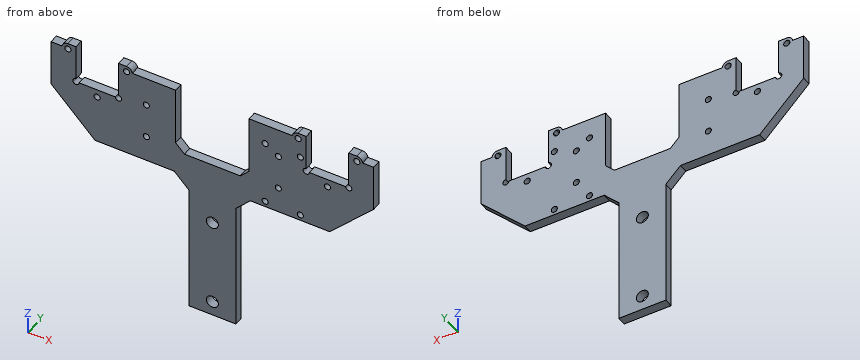
from build123d import *

# Parameters (mm, degrees)
EXTRUDE_6_DEPTH         = 3
HOLE_WIZARD_4_1_4_1_1_D = 4.1
HOLE_WIZARD_2_1_2_1_1_D = 2.1
EXTRUDE_START           = -3
SKETCH_39_R             = 1.05
EXTRUDE_7_DEPTH         = 3
HOLE_WIZARD_2_1_2_1_2_D = 2.1
CHAMFER_3_SIZE          = 3


with BuildPart() as part:
    # 草图33 → 凸台-拉伸6 (new body)
    with BuildSketch(Plane(origin=(0, 0, 0), x_dir=(1, 0, 0), z_dir=(0, 1, 0))):
        Polygon((110, 16), (110, 0), (101.5, 0), (101.5, 11.5), (87, 11.5), (87, 0), (67.5, 0), (67.5, 23), (42.5, 23), (42.5, 0), (23, 0), (23, 11.5), (8.5, 11.5), (8.5, 0), (0, 0), (0, 16), (15, 31), (42, 31), (47, 36), (47, 80), (63, 80), (63, 36), (68, 31), (95, 31), align=None)
    extrude(amount=EXTRUDE_6_DEPTH)

    # Ø4.1 (4.1) 直径孔1 (through all)
    with Locations(Plane(origin=(0, 3, 0), x_dir=(1, 0, 0), z_dir=(0, 1, 0))):
        with Locations((55, 75), (55, 45)):
            Hole(HOLE_WIZARD_4_1_4_1_1_D / 2)

    # Ø2.1 (2.1) 直径孔1 (through all)
    with Locations(Plane(origin=(0, 3, 0), x_dir=(1, 0, 0), z_dir=(0, 1, 0))):
        with Locations((32.5, 10), (5.75, 0.25), (15.75, 14.25), (25.75, 0.25), (94.25, 14.25), (104.25, 0.25), (84.25, 0.25), (73, 29), (85, 7), (73, 7), (85, 29), (32.5, 22), (77.5, 22), (77.5, 10)):
            Hole(HOLE_WIZARD_2_1_2_1_1_D / 2)

    # 草图39 → 凸台-拉伸7 (add)
    # profile 1 of 4: a face of its own
    with BuildSketch(Plane(origin=(0, 3, 0), x_dir=(1, 0, 0), z_dir=(0, 1, 0)).offset(EXTRUDE_START)):
        with BuildLine():
            Line((5.75, -1.75), (8.5, -1.75))
            Line((8.5, -1.75), (8.5, 0))
            Line((8.5, 0), (7.734313483, 0))
            ThreePointArc((7.734313483, 0), (4.427124344, 1.75), (5.75, -1.75))
        make_face()
        with Locations(Location((5.75, 0.25, 0), (0, 0, 270))):
            Circle(SKETCH_39_R, mode=Mode.SUBTRACT)
    # profile 2 of 4: a face of its own
    with BuildSketch(Plane(origin=(0, 3, 0), x_dir=(1, 0, 0), z_dir=(0, 1, 0)).offset(EXTRUDE_START)):
        with BuildLine():
            Line((25.75, -1.75), (23, -1.75))
            Line((23, -1.75), (23, 0))
            Line((23, 0), (23.765686517, 0))
            ThreePointArc((23.765686517, 0), (27.072875656, 1.75), (25.75, -1.75))
        make_face()
        with Locations(Location((25.75, 0.25, 0), (0, 0, 270))):
            Circle(SKETCH_39_R, mode=Mode.SUBTRACT)
    # profile 3 of 4: a face of its own
    with BuildSketch(Plane(origin=(0, 3, 0), x_dir=(1, 0, 0), z_dir=(0, 1, 0)).offset(EXTRUDE_START)):
        with BuildLine():
            Line((101.5, 0), (102.265686517, 0))
            ThreePointArc((102.265686517, 0), (105.572875656, 1.75), (104.25, -1.75))
            Line((104.25, -1.75), (101.5, -1.75))
            Line((101.5, -1.75), (101.5, 0))
        make_face()
        with Locations(Location((104.25, 0.25, 0), (0, 0, 270))):
            Circle(SKETCH_39_R, mode=Mode.SUBTRACT)
    # profile 4 of 4: a face of its own
    with BuildSketch(Plane(origin=(0, 3, 0), x_dir=(1, 0, 0), z_dir=(0, 1, 0)).offset(EXTRUDE_START)):
        with BuildLine():
            Line((84.25, -1.75), (87, -1.75))
            Line((87, -1.75), (87, 0))
            Line((87, 0), (86.234313483, 0))
            ThreePointArc((86.234313483, 0), (82.927124344, 1.75), (84.25, -1.75))
        make_face()
        with Locations(Location((84.25, 0.25, 0), (0, 0, 270))):
            Circle(SKETCH_39_R, mode=Mode.SUBTRACT)
    extrude(amount=EXTRUDE_7_DEPTH)

    # Ø2.1 (2.1) 直径孔2 (through all)
    with Locations(Plane(origin=(0, 3, 0), x_dir=(1, 0, 0), z_dir=(0, 1, 0))):
        with Locations((8.5, 11.5), (23, 11.5), (87, 11.5), (101.5, 11.5)):
            Hole(HOLE_WIZARD_2_1_2_1_2_D / 2)

    # 倒角3
    chamfer_3_edges = [part.edges().sort_by_distance(p)[0] for p in [
        (67.5, 1.5, -23),
        (42.5, 1.5, -23),
    ]]
    chamfer(chamfer_3_edges, length=CHAMFER_3_SIZE)


solid = part.part
Could you check a few things on this model? Use its own coordinates, in mm. Give positions to 0.01 mm unless a question says otherwise; leave off trailing zeros. Order: outer loops, then holes, each group sorted by start corner. A loop starts at its lowest first (then second) coordinate and runs counter-clockwise, first axis right, second up.
1. Suppose I cut it at C-C (x = 66). Write out the boundary of the cut face in (y, z), plus the area to 3 significant figures.
Answers below:
outline: (0, -33) - (3, -33) - (3, -21.5) - (0, -21.5) - close
area: 34.5 mm2
2. Suppose I cut it at A-A (z = -45). Write out the boundary of the cut face in (x, y).
Answers below:
outline: (47, 0) - (52.95, 0) - (52.95, 3) - (47, 3) - close; (57.05, 0) - (63, 0) - (63, 3) - (57.05, 3) - close
3. For pin 1 (1.5 mm diameter, centred on y = 2, z = -65.5, fed in from +X); pin 2 (1.7 mm diameter, centred on x = 15.75, z = -14.25, fed in from -Y); pin 3 (0.9 mm diameter, centred on x = 17, y = 1, fed in from +Z); pin 4 (1 mm diameter, centred on x = 49.5, y = 1.5, fed in from +Z), each with a flat end and sliding along its axis, tell me the tip position at first contact or that it passes through.
Answers below:
pin 1: stops at x = 63
pin 2: passes through
pin 3: stops at z = -11.5
pin 4: stops at z = -23
4. I need wall thicknesses on L1, parallel to X at y = 2, z = -7; L2, parallel to Z at x = 73, y = 0.85; L3, parallel to X at y = 1.65, z = -10. Which ranges of each line are inside material? Lowest first, please.
Answers below:
L1: x = 0 to 8.5, 23 to 42.5, 67.5 to 71.95, 74.05 to 83.95, 86.05 to 87, 101.5 to 110
L2: z = -31 to -30.05, -27.95 to -8.05, -5.95 to 0
L3: x = 0 to 8.5, 23 to 31.45, 33.55 to 42.5, 67.5 to 76.45, 78.55 to 87, 101.5 to 110
5. Suppose I cut it at B-B (y = 0.85). State how many separate pieces and enclosed holes the cut face has, plus the area to 3 significant figures.
Answers below:
separate pieces: 1
enclosed holes: 16
area: 3,040 mm2
6. Suppose I cut it at D-D (z = -54). Write out the boundary of the cut face in (x, y), plus the area to 3 significant figures.
Answers below:
outline: (47, 0) - (63, 0) - (63, 3) - (47, 3) - close
area: 48.0 mm2
